Part model, mm, in its own coordinate system. A direction names the side the tool comes from. Give positions to 0.01 mm unless a question says otherwise; leave off trailing zeros. Write each loop counter-clockwise with the first axis right and the second up, starting at its lowest first coordinate (ties: lowest second). Pieces come first, ordered by that corner, then holes. Notation, with made-up numbers: M 4,-30 L 10,-30 A26 cw 10,-11 Z; hole C -33,-8 d10. An arc over 180 degrees is marked long. Answer as CSV lines item,"result". Start each with the question number.
Item 1: Band-saw the part on B-B, the plane x = 46. List the corners of the cut face in (y, z), then the cut area to 3 significant figures.
Item 2: Two-plate mould, pull along Y, no slides. Class faces 4 (the cylindrical face through (24, -2, 9)), 5 (the cylindrical face through (9, 23, 1)), 6 (the flat face through (53.6, -1, 7)): +Y half, -Y half, draft (parallel to the pull), parting line (faces both ways), or undercut.
Item 3: Band-saw the part on A-A, the plane x = 28.5. List the corners of the cut face in (y, z), then the cut area to 3 significant figures.
Item 4: Pin check, flat tips, straight feed: pin 1 (6 mm diameter, centred on x = 48.5, y = 23, fed in from -Z); pin 2 (0.5 mm diameter, centred on x = 9.5, y = 66, fed in from -Z); pin 3 (3 mm diameter, centred on x = 9, y = 24, fed in from +Z). Stop position of each tip, or through.
Item 5: 3-axis set-ups, long thin cutter, end or side, ignore diameter. For faces 1 (the flat face through (61, 29.25, 7)), 2 (the cylindrical face through (62, 3, 9)), 3 (the flat face through (30, 85.5, 5)): which of +Z, -Z, +X, -X, +Y, -Y reach the whole face in a straight line?
Item 6: Wall check: L1, parallel to Y at x = 9, z = 0.7; L2, parallel to Y at x = 4, z = 5; L3, parallel to Y at x = 30, z = 4.75. Give the ranges that are in metal, low to high. Write a range as from..to.
from build123d import *

# Parameters (mm, degrees)
TOP_PLATE_DEPTH                = 2
WALL_OUTER_HALF_DEPTH          = 10
WALL_INNER_HALF_DEPTH          = 9
LENS_FACE_ROUND_OVER_R         = 2.5
SKETCH_4_R                     = 8
SKETCH_4_R_2                   = 5
LENS_BEZEL_RING_DEPTH          = 1.5
SKETCH_5_R                     = 2.3
CORNER_POSTS_DEPTH             = 10
POST_START                     = 10
SKETCH_6_R                     = 0.8
POST_PILOT_HOLES_M2_DEPTH      = 7
SKETCH_7_W                     = 12
SKETCH_7_H                     = 1
GRIP_GROOVES_DEPTH             = 0.6
SKETCH_8_R                     = 1
BOOT_RESET_PINHOLES_DEPTH      = 108.993055471
SKETCH_9_W                     = 6
SKETCH_9_H                     = 4.2
SHUTTER_WINDOW_DEPTH           = 108.993055471
SKETCH_10_R                    = 5
LENS_HOLE_DEPTH                = 108.993055471
SKETCH_11_R                    = 0.75
LED_LIGHT_HOLES_D1_D4_D5_DEPTH = 108.993055471
USB_C_START                    = 59
SKETCH_12_W                    = 4.2
SKETCH_12_H                    = 10.5
USB_C_WINDOW_DEPTH             = 4.5
POWER_START                    = 59
SKETCH_13_W                    = 4.5
SKETCH_13_H                    = 8
POWER_SWITCH_SLOT_DEPTH        = 4.5
SWITCH_START                   = 61.5
SKETCH_14_W                    = 6
SKETCH_14_H                    = 12
SWITCH_FINGER_POCKET_DEPTH     = 1.5


with BuildPart() as part:
    # 草圖1 → top plate (new body)
    with BuildSketch(Plane.XY):
        with BuildLine():
            Line((2, -2.5), (58, -2.5))
            ThreePointArc((58, -2.5), (61.181980515, -1.181980515), (62.5, 2))
            Line((62.5, 2), (62.5, 83))
            ThreePointArc((62.5, 83), (61.181980515, 86.181980515), (58, 87.5))
            Line((58, 87.5), (2, 87.5))
            ThreePointArc((2, 87.5), (-1.181980515, 86.181980515), (-2.5, 83))
            Line((-2.5, 83), (-2.5, 2))
            ThreePointArc((-2.5, 2), (-1.181980515, -1.181980515), (2, -2.5))
        make_face()
    extrude(amount=TOP_PLATE_DEPTH)

    # 草圖2 → wall outer half (add)
    with BuildSketch(Plane.XY):
        with BuildLine():
            Line((2, -2.5), (58, -2.5))
            ThreePointArc((58, -2.5), (61.181980515, -1.181980515), (62.5, 2))
            Line((62.5, 2), (62.5, 83))
            ThreePointArc((62.5, 83), (61.181980515, 86.181980515), (58, 87.5))
            Line((58, 87.5), (2, 87.5))
            ThreePointArc((2, 87.5), (-1.181980515, 86.181980515), (-2.5, 83))
            Line((-2.5, 83), (-2.5, 2))
            ThreePointArc((-2.5, 2), (-1.181980515, -1.181980515), (2, -2.5))
        make_face()
        with BuildLine():
            Line((2, -1.5), (58, -1.5))
            ThreePointArc((58, -1.5), (60.474873734, -0.474873734), (61.5, 2))
            Line((61.5, 2), (61.5, 83))
            ThreePointArc((61.5, 83), (60.474873734, 85.474873734), (58, 86.5))
            Line((58, 86.5), (2, 86.5))
            ThreePointArc((2, 86.5), (-0.474873734, 85.474873734), (-1.5, 83))
            Line((-1.5, 83), (-1.5, 2))
            ThreePointArc((-1.5, 2), (-0.474873734, -0.474873734), (2, -1.5))
        make_face(mode=Mode.SUBTRACT)
    extrude(amount=WALL_OUTER_HALF_DEPTH)

    # 草圖3 → wall inner half (add)
    with BuildSketch(Plane.XY):
        with BuildLine():
            Line((2, -1.5), (58, -1.5))
            ThreePointArc((58, -1.5), (60.474873734, -0.474873734), (61.5, 2))
            Line((61.5, 2), (61.5, 83))
            ThreePointArc((61.5, 83), (60.474873734, 85.474873734), (58, 86.5))
            Line((58, 86.5), (2, 86.5))
            ThreePointArc((2, 86.5), (-0.474873734, 85.474873734), (-1.5, 83))
            Line((-1.5, 83), (-1.5, 2))
            ThreePointArc((-1.5, 2), (-0.474873734, -0.474873734), (2, -1.5))
        make_face()
        with BuildLine():
            Line((2, -0.5), (58, -0.5))
            ThreePointArc((58, -0.5), (59.767766953, 0.232233047), (60.5, 2))
            Line((60.5, 2), (60.5, 83))
            ThreePointArc((60.5, 83), (59.767766953, 84.767766953), (58, 85.5))
            Line((58, 85.5), (2, 85.5))
            ThreePointArc((2, 85.5), (0.232233047, 84.767766953), (-0.5, 83))
            Line((-0.5, 83), (-0.5, 2))
            ThreePointArc((-0.5, 2), (0.232233047, 0.232233047), (2, -0.5))
        make_face(mode=Mode.SUBTRACT)
    extrude(amount=WALL_INNER_HALF_DEPTH)

    # lens face round-over
    # the kernel refuses this fillet: 2.5 mm, written as the material it takes off along each edge
    with BuildSketch(Plane(origin=(2, 2, 10), x_dir=(-1, 0, 0), z_dir=(0, 1, 0))) as lens_face_round_over_piece_1:
        with BuildLine():
            CenterArc((4.5 - LENS_FACE_ROUND_OVER_R, -LENS_FACE_ROUND_OVER_R), LENS_FACE_ROUND_OVER_R, 0, 90)
            Line((4.5 - LENS_FACE_ROUND_OVER_R, 0), (4.5, 0))
            Line((4.5, 0), (4.5, -LENS_FACE_ROUND_OVER_R))
        make_face()
    revolve(axis=Axis((2, 2, 10), (0, 0, 1)), revolution_arc=90, mode=Mode.SUBTRACT)
    with BuildSketch(Plane(origin=(-2.5, 83, 10), x_dir=(1, 0, 0), z_dir=(0, -1, 0)), Plane(origin=(62.5, 2, 10), x_dir=(-1, 0, 0), z_dir=(0, 1, 0))) as lens_face_round_over_piece_2:
        with BuildLine():
            CenterArc((LENS_FACE_ROUND_OVER_R, -LENS_FACE_ROUND_OVER_R), LENS_FACE_ROUND_OVER_R, 90, 90)
            Line((0, -LENS_FACE_ROUND_OVER_R), (0, 0))
            Line((0, 0), (LENS_FACE_ROUND_OVER_R, 0))
        make_face()
    extrude(amount=81, mode=Mode.SUBTRACT)
    with BuildSketch(Plane(origin=(2, 83, 10), x_dir=(0, 1, 0), z_dir=(1, 0, 0))) as lens_face_round_over_piece_3:
        with BuildLine():
            CenterArc((4.5 - LENS_FACE_ROUND_OVER_R, -LENS_FACE_ROUND_OVER_R), LENS_FACE_ROUND_OVER_R, 0, 90)
            Line((4.5, -LENS_FACE_ROUND_OVER_R), (4.5, 0))
            Line((4.5, 0), (4.5 - LENS_FACE_ROUND_OVER_R, 0))
        make_face()
    revolve(axis=Axis((2, 83, 10), (0, 0, 1)), revolution_arc=90, mode=Mode.SUBTRACT)
    with BuildSketch(Plane(origin=(58, 87.5, 10), x_dir=(0, -1, 0), z_dir=(-1, 0, 0))) as lens_face_round_over_piece_4:
        with BuildLine():
            CenterArc((LENS_FACE_ROUND_OVER_R, -LENS_FACE_ROUND_OVER_R), LENS_FACE_ROUND_OVER_R, 90, 90)
            Line((0, -LENS_FACE_ROUND_OVER_R), (0, 0))
            Line((0, 0), (LENS_FACE_ROUND_OVER_R, 0))
        make_face()
    extrude(amount=56, mode=Mode.SUBTRACT)
    with BuildSketch(Plane(origin=(58, 83, 10), x_dir=(1, 0, 0), z_dir=(0, -1, 0))) as lens_face_round_over_piece_5:
        with BuildLine():
            CenterArc((4.5 - LENS_FACE_ROUND_OVER_R, -LENS_FACE_ROUND_OVER_R), LENS_FACE_ROUND_OVER_R, 0, 90)
            Line((4.5, -LENS_FACE_ROUND_OVER_R), (4.5, 0))
            Line((4.5, 0), (4.5 - LENS_FACE_ROUND_OVER_R, 0))
        make_face()
    revolve(axis=Axis((58, 83, 10), (0, 0, 1)), revolution_arc=90, mode=Mode.SUBTRACT)
    with BuildSketch(Plane(origin=(58, 2, 10), x_dir=(0, -1, 0), z_dir=(-1, 0, 0))) as lens_face_round_over_piece_6:
        with BuildLine():
            CenterArc((4.5 - LENS_FACE_ROUND_OVER_R, -LENS_FACE_ROUND_OVER_R), LENS_FACE_ROUND_OVER_R, 0, 90)
            Line((4.5, -LENS_FACE_ROUND_OVER_R), (4.5, 0))
            Line((4.5, 0), (4.5 - LENS_FACE_ROUND_OVER_R, 0))
        make_face()
    revolve(axis=Axis((58, 2, 10), (0, 0, 1)), revolution_arc=90, mode=Mode.SUBTRACT)
    with BuildSketch(Plane(origin=(2, -2.5, 10), x_dir=(0, 0, -1), z_dir=(1, 0, 0))) as lens_face_round_over_piece_7:
        with BuildLine():
            CenterArc((LENS_FACE_ROUND_OVER_R, LENS_FACE_ROUND_OVER_R), LENS_FACE_ROUND_OVER_R, 180, 90)
            Line((0, LENS_FACE_ROUND_OVER_R), (0, 0))
            Line((0, 0), (LENS_FACE_ROUND_OVER_R, 0))
        make_face()
    extrude(amount=56, mode=Mode.SUBTRACT)

    # 草圖4 → lens bezel ring (add)
    with BuildSketch(Plane.XY):
        with Locations((30, 25)):
            Circle(SKETCH_4_R)
        with Locations((30, 25)):
            Circle(SKETCH_4_R_2, mode=Mode.SUBTRACT)
    extrude(amount=-LENS_BEZEL_RING_DEPTH)

    # 草圖5 → corner posts (add)
    with BuildSketch(Plane.XY):
        with Locations((4, 4)):
            Circle(SKETCH_5_R)
        with Locations((56, 4)):
            Circle(SKETCH_5_R)
        with Locations((4, 71)):
            Circle(SKETCH_5_R)
        with Locations((56, 71)):
            Circle(SKETCH_5_R)
    extrude(amount=CORNER_POSTS_DEPTH)

    # 草圖6 → post pilot holes M2 (cut)
    with BuildSketch(Plane.XY.offset(POST_START)):
        with Locations((4, 4)):
            Circle(SKETCH_6_R)
        with Locations((56, 4)):
            Circle(SKETCH_6_R)
        with Locations((4, 71)):
            Circle(SKETCH_6_R)
        with Locations((56, 71)):
            Circle(SKETCH_6_R)
    extrude(amount=-POST_PILOT_HOLES_M2_DEPTH, mode=Mode.SUBTRACT)

    # 草圖7 → grip grooves (cut)
    with BuildSketch(Plane.XY):
        with Locations((9.5, 50)):
            Rectangle(SKETCH_7_W, SKETCH_7_H)
        with Locations((9.5, 54)):
            Rectangle(SKETCH_7_W, SKETCH_7_H)
        with Locations((9.5, 58)):
            Rectangle(SKETCH_7_W, SKETCH_7_H)
        with Locations((9.5, 62)):
            Rectangle(SKETCH_7_W, SKETCH_7_H)
        with Locations((9.5, 66)):
            Rectangle(SKETCH_7_W, SKETCH_7_H)
        with Locations((9.5, 70)):
            Rectangle(SKETCH_7_W, SKETCH_7_H)
    extrude(amount=GRIP_GROOVES_DEPTH, mode=Mode.SUBTRACT)

    # 草圖8 → BOOT/RESET pinholes (cut, through all)
    with BuildSketch(Plane.XY):
        with Locations((9, 24)):
            Circle(SKETCH_8_R)
        with Locations((9, 32)):
            Circle(SKETCH_8_R)
    extrude(amount=BOOT_RESET_PINHOLES_DEPTH, mode=Mode.SUBTRACT)

    # 草圖9 → shutter window (cut, through all)
    with BuildSketch(Plane(origin=(0, 0, 0), x_dir=(1, 0, 0), z_dir=(0, 1, 0))):
        with Locations((50.6, -7.7)):
            Rectangle(SKETCH_9_W, SKETCH_9_H)
    extrude(amount=-SHUTTER_WINDOW_DEPTH, mode=Mode.SUBTRACT)

    # 草圖10 → lens hole (cut, through all)
    with BuildSketch(Plane.XY):
        with Locations((30, 25)):
            Circle(SKETCH_10_R)
    extrude(amount=LENS_HOLE_DEPTH, mode=Mode.SUBTRACT)

    # 草圖11 → LED light holes D1 D4 D5 (cut, through all)
    with BuildSketch(Plane.XY):
        with Locations((14, 4.5)):
            Circle(SKETCH_11_R)
        with Locations((9, 4.5)):
            Circle(SKETCH_11_R)
        with Locations((53, 11.2)):
            Circle(SKETCH_11_R)
    extrude(amount=LED_LIGHT_HOLES_D1_D4_D5_DEPTH, mode=Mode.SUBTRACT)

    # 草圖12 → USB-C window (cut)
    with BuildSketch(Plane(origin=(0, 0, 0), x_dir=(0, 0, -1), z_dir=(1, 0, 0)).offset(USB_C_START)):
        with Locations((-7.9, 24)):
            Rectangle(SKETCH_12_W, SKETCH_12_H)
    extrude(amount=USB_C_WINDOW_DEPTH, mode=Mode.SUBTRACT)

    # 草圖13 → power switch slot (cut)
    with BuildSketch(Plane(origin=(0, 0, 0), x_dir=(0, 0, -1), z_dir=(1, 0, 0)).offset(POWER_START)):
        with Locations((-7.75, 11)):
            Rectangle(SKETCH_13_W, SKETCH_13_H)
    extrude(amount=POWER_SWITCH_SLOT_DEPTH, mode=Mode.SUBTRACT)

    # 草圖14 → switch finger pocket (cut)
    with BuildSketch(Plane(origin=(0, 0, 0), x_dir=(0, 0, -1), z_dir=(1, 0, 0)).offset(SWITCH_START)):
        with Locations((-7, 11)):
            Rectangle(SKETCH_14_W, SKETCH_14_H)
    extrude(amount=SWITCH_FINGER_POCKET_DEPTH, mode=Mode.SUBTRACT)


solid = part.part
Output:
1,outline,"M -2.5,0 L 87.5,0 L 87.5,7.5 A2.5 ccw 86.5,9.5 L 86.5,9 L 85.5,9 L 85.5,2 L -0.5,2 L -0.5,9 L -1.5,9 L -1.5,9.5 A2.5 ccw -2.5,7.5 Z"
1,area,"208 mm²"
2,face 4,"-Y half"
2,face 5,"undercut"
2,face 6,"draft"
3,outline,"M -2.5,0 L 17.14,0 L 17.14,-1.5 L 20.23,-1.5 L 20.23,2 L -0.5,2 L -0.5,9 L -1.5,9 L -1.5,9.5 A2.5 ccw -2.5,7.5 Z; M 29.77,-1.5 L 32.86,-1.5 L 32.86,0 L 87.5,0 L 87.5,7.5 A2.5 ccw 86.5,9.5 L 86.5,9 L 85.5,9 L 85.5,2 L 29.77,2 Z"
3,area,"198 mm²"
4,pin 1,"z = 0"
4,pin 2,"z = 0.6"
4,pin 3,"z = 2"
5,face 1,"+Z, +X"
5,face 2,"+Z, +X, +Y, -Y"
5,face 3,"+Z"
6,L1,"-2.5..3.75, 5.25..23, 25..31, 33..87.5"
6,L2,"-2.5..-0.5, 1.7..3.2, 4.8..6.3, 68.7..70.2, 71.8..73.3, 85.5..87.5"
6,L3,"-2.5..-0.5, 85.5..87.5"
